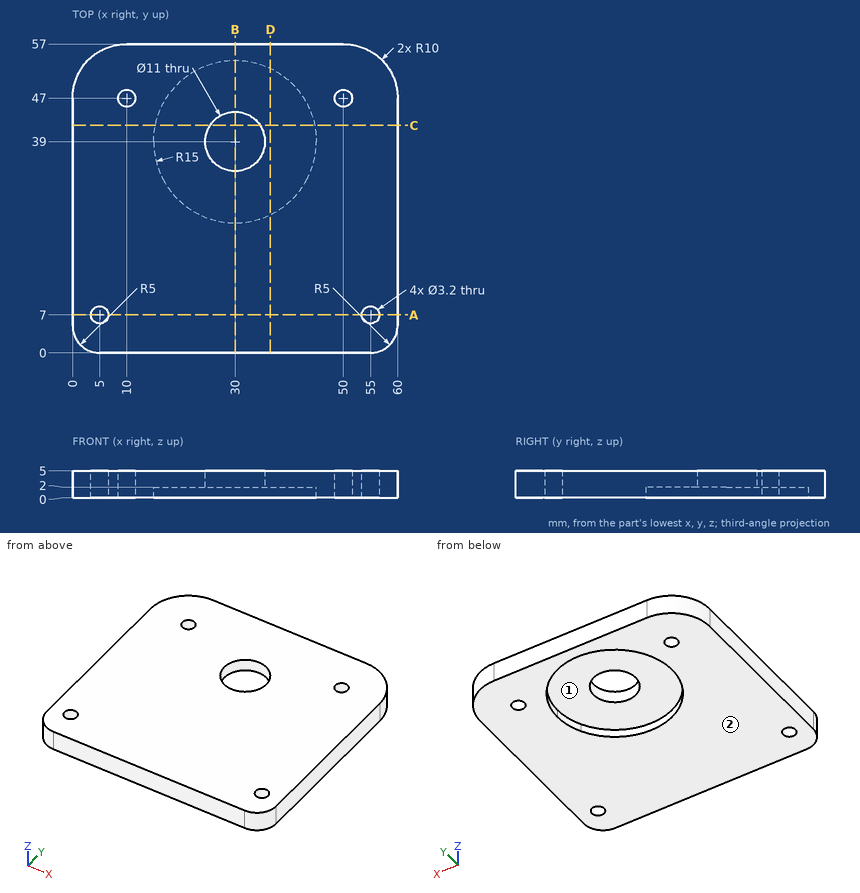
Job drawing, mm, ordinate dimensions from the low corner. One solid piece. A direction names the side the tool comes from. Round coordinates to 2 decimals unless told otherwise and drop trailing zeros. Loops run counter-clockwise (first coordinate to the right, second up) from the corner with the lowest first, then second, coordinate; pieces in that order, holes last. Notation, with made-up numbers: (31.25, 83) -> (87.25, 83) arc R29 ccw to (87.25, 107) -> close; hole circle Ø9 at (-21.75, -28.5). An arc over 180 degrees is marked (long way). Use a Markdown table: item, result.
1) Cut at C-C, the plane y = 42. List the corners of the cut face in (x, z).
The answers:
| item | result |
|---|---|
| outline | (0, 0) -> (15.3, 0) -> (15.3, 2) -> (25.39, 2) -> (25.39, 5) -> (0, 5) -> close; (34.61, 2) -> (44.7, 2) -> (44.7, 0) -> (60, 0) -> (60, 5) -> (34.61, 5) -> close |
2) Cut at B-B, the plane x = 30. List the corners of the cut face in (y, z), and give its area (3 significant figures).
The answers:
| item | result |
|---|---|
| outline | (0, 0) -> (24, 0) -> (24, 2) -> (33.5, 2) -> (33.5, 5) -> (0, 5) -> close; (44.5, 2) -> (54, 2) -> (54, 0) -> (57, 0) -> (57, 5) -> (44.5, 5) -> close |
| area | 192 mm2 |
3) Cut at A-A, the plane y = 7. List the corners of the cut face in (x, z), and give its area (3 significant figures).
The answers:
| item | result |
|---|---|
| outline | (0, 0) -> (3.4, 0) -> (3.4, 5) -> (0, 5) -> close; (6.6, 0) -> (53.4, 0) -> (53.4, 5) -> (6.6, 5) -> close; (56.6, 0) -> (60, 0) -> (60, 5) -> (56.6, 5) -> close |
| area | 268 mm2 |
4) Cut at D-D, the plane x = 36.5. List the corners of the cut face in (y, z).
The answers:
| item | result |
|---|---|
| outline | (0, 0) -> (25.48, 0) -> (25.48, 2) -> (52.52, 2) -> (52.52, 0) -> (57, 0) -> (57, 5) -> (0, 5) -> close |
5) Drop flat-ended pins along their axis: pin 1 Ø1.9 at (x, y) = (50, 47) entering from -Z; pin 2 Ø15 at (x, y) = (24, 35) entering from -Z. Give the stop position or say it passes through.
The answers:
| item | result |
|---|---|
| pin 1 | passes through |
| pin 2 | stops at z = 2 |
6) Tool access for the marked faces 1 and 2: list every direction of +Z, -Z, +X, -X, +Y, -Y with a clear straight run to the whole face (end or side of a thin tool).
The answers:
| item | result |
|---|---|
| face 1 | -Z |
| face 2 | -Z, +X, -X, +Y, -Y |
7) Probe line 1 (Z direction, x = 38, y = 38); line 2 (Y direction, x = 10, z = 2.45); line 3 (Y direction, x = 30, z = 3.4). List the from-to ranges inside material, lowest first. Write a range as [from, to].
The answers:
| item | result |
|---|---|
| line 1 | z = [2, 5] |
| line 2 | y = [0, 45.4], [48.6, 57] |
| line 3 | y = [0, 33.5], [44.5, 57] |
